Geometry check sheet. Reference: the model listing, model coordinates, mm. A direction names the side the tool comes from. Coordinates: 2 decimals unless noted, no trailing zeros. Order: outer loops, then holes, each group sorted by start corner. A loop starts at its lowest first (then second) coordinate and runs counter-clockwise, first axis right, second up. Notation, with made-up numbers: (-1.5, 61) - (39.5, 61) arc R18 cw to (39.5, 95) - close; hole circle Ø3 at (-36, 73.5). An arc over 180 degrees is marked (long way). Return JSON: item names as keys, results as strings. Group by question number.
Item 1: Draft check along Z on faces 1 (the flat face through (-1, -18.7, 15.3)), 2 (the flat face through (-3, -21, 15)), 3 (the cylindrical face through (19.783, -0.221, 28.686)). Enter one of: pulls with the +Z half, pulls with the -Z half, needs draft (parallel to the pull), parting line crosses it, or undercut.
Item 2: Section check B-B on x = 9. Enter the section's corners in (y, z), then the cut area to 3 significant figures.
Item 3: Section check A-A on z = 7.5. Enter the section's corners in (x, y), then the cut area to 3 significant figures.
Item 4: Section check C-C on y = 0. Enter the section's corners in (x, z).
Item 5: Tool access check on faces 4 (the flat face through (-13, -11, 37)), 5 (the flat face through (18.6, -5.6, 18.6)), 6 (the flat face through (1, -18.7, 15.3)), 7 (the cylindrical face through (19.783, -7.221, 21.686)), 8 (the flat face through (5, -25, 6)). Record the directions out of +Z, -Z, +X, -X, +Y, -Y that give a thin tool (end or side, any length) a straight path to the whole face; none if there is none.
Item 6: Gauge pin test, flat ends, axial feed: pin 1 (1 mm diameter, centred on x = -8, z = 9.5, fed in from +Y); pin 2 (3 mm diameter, centred on y = -24.5, z = 8.5, fed in from -X); pin 3 (3 mm diameter, centred on y = 1, z = 25.5, fed in from -X); pin 4 (6 mm diameter, centred on x = -13, y = -17, fed in from +Z). Record the tip position at first contact, or that the pin passes through.
Item 7: Scan lines: probe 1 along Y at (x, z) = (15, 13); probe 2 along Y at (x, z) = (14, 24); probe 3 along X at (y, z) = (1.5, 30). Record each from-to range of solid material in increasing order.
Item 8: Section check D-D on x = 2.5. Enter the section's corners in (y, z), then the cut area to 3 significant figures.
from build123d import *

# Parameters (mm, degrees)
BOSS_EXTRUDE1_DEPTH      = 40
EXTRUDE_START            = -25
SKETCH_5_W               = 10
SKETCH_5_H               = 28
EXTRUDE_2_DEPTH          = 15
CUT_EXTRUDE1_DEPTH       = 53.39274759
CUT_EXTRUDE1_DEPTH_BACK  = 53.39274759
SKETCH2_R                = 15
SKETCH5_R                = 11
CUT_EXTRUDE3_DEPTH       = 10
SKETCH7_W                = 6.152946469
SKETCH7_H                = 22
CUT_EXTRUDE9_DEPTH       = 10
SKETCH_2_W               = 5
SKETCH_2_H               = 14
CUT_EXTRUDE_2_DEPTH      = 20
CUT_EXTRUDE_6_DEPTH      = 51.368641203
CUT_EXTRUDE_6_DEPTH_BACK = 51.368641203
SKETCH_7_R               = 1.85
SKETCH6_W                = 2
SKETCH6_H                = 28
CUT_EXTRUDE8_DEPTH       = 53.392747702
CUT_EXTRUDE10_REACH      = 63.871
SKETCH8_R                = 3
CUT_EXTRUDE11_REACH      = 61.843
SKETCH13_R               = 3.25
SKETCH14_W               = 40
SKETCH14_H               = 38
SKETCH14_R               = 3
SKETCH14_R_2             = 1.7
BOSS_EXTRUDE2_DEPTH      = 2
CIRPATTERN1_START        = 10
CIRPATTERN1_OUTLINE_R    = 3.25
CIRPATTERN1_DEPTH        = 8.6
CIRPATTERN1_START_2      = 18.6
CIRPATTERN1_2_OUTLINE_R  = 1.7
CIRPATTERN1_2_DEPTH      = 2.4
CIRPATTERN2_START        = 15.6
CIRPATTERN2_OUTLINE_R    = 3.25
CIRPATTERN2_DEPTH        = 3
CIRPATTERN2_START_2      = 18.6
CIRPATTERN2_2_OUTLINE_R  = 1.7
CIRPATTERN2_2_DEPTH      = 2.4
CHAMFER1_SIZE            = 4


with BuildPart() as part:
    # Sketch1 → Boss-Extrude1 (new body)
    with BuildSketch(Plane.XY):
        with BuildLine():
            Line((0, 19), (19, 19))
            Line((19, 19), (19, -19))
            Line((19, -19), (0, -19))
            ThreePointArc((0, -19), (-19, 0), (0, 19))
        make_face()
    extrude(amount=BOSS_EXTRUDE1_DEPTH)

    # 草圖5 → 填料-伸長2 (add)
    with BuildSketch(Plane.XY.offset(40).offset(EXTRUDE_START)):
        with Locations((0, -14)):
            Rectangle(SKETCH_5_W, SKETCH_5_H)
    extrude(amount=-EXTRUDE_2_DEPTH)

    # Sketch2 → Cut-Extrude1 (cut, two sides: drawn at the far end of the back side and taken through both)
    with BuildSketch(Plane.XY.offset(40).offset(-CUT_EXTRUDE1_DEPTH_BACK)):
        Circle(SKETCH2_R)
    extrude(amount=CUT_EXTRUDE1_DEPTH + CUT_EXTRUDE1_DEPTH_BACK, mode=Mode.SUBTRACT)

    # Sketch5 → Cut-Extrude3 (cut)
    with BuildSketch(Plane(origin=(-19, 0, 0), x_dir=(0, 1, 0), z_dir=(-1, 0, 0))):
        with Locations((0, -34)):
            Circle(SKETCH5_R)
    extrude(amount=-CUT_EXTRUDE3_DEPTH, mode=Mode.SUBTRACT)

    # Sketch7 → Cut-Extrude9 (cut)
    with BuildSketch(Plane.ZY.offset(19)):
        with Locations((37.076473234, 0)):
            Rectangle(SKETCH7_W, SKETCH7_H)
    extrude(amount=-CUT_EXTRUDE9_DEPTH, mode=Mode.SUBTRACT)

    # 草圖2 → 除料-伸長2 (cut)
    with BuildSketch(Plane.XY.offset(40)):
        with Locations((13.1, 0)):
            Rectangle(SKETCH_2_W, SKETCH_2_H)
    extrude(amount=-CUT_EXTRUDE_2_DEPTH, mode=Mode.SUBTRACT)

    # 草圖7 → 除料-伸長6 (cut, two sides: drawn at the far end of the back side and taken through both)
    with BuildSketch(Plane(origin=(0, -5, 0), x_dir=(0, 0, 1), z_dir=(-1, 0, 0)).offset(-CUT_EXTRUDE_6_DEPTH_BACK)):
        with Locations(Location((7.5, -18, 0), (0, 0, 90))):
            Circle(SKETCH_7_R)
    extrude(amount=CUT_EXTRUDE_6_DEPTH + CUT_EXTRUDE_6_DEPTH_BACK, mode=Mode.SUBTRACT)

    # Sketch6 → Cut-Extrude8 (cut, through all)
    with BuildSketch(Plane.XY):
        with Locations((0, -14)):
            Rectangle(SKETCH6_W, SKETCH6_H)
    extrude(amount=CUT_EXTRUDE8_DEPTH, mode=Mode.SUBTRACT)

    # Sketch8 → Cut-Extrude10 (cut, up to next)
    with BuildSketch(Plane(origin=(19, 0, 0), x_dir=(0, 0, -1), z_dir=(1, 0, 0)), mode=Mode.PRIVATE) as cut_extrude10_sk1:
        with Locations((-20, 0)):
            Circle(SKETCH8_R)
    cut_extrude10_tool1 = extrude(cut_extrude10_sk1.sketch, amount=-CUT_EXTRUDE10_REACH, mode=Mode.PRIVATE) & part.part
    add(cut_extrude10_tool1.solids().sort_by_distance((19, 0, 20))[0], mode=Mode.SUBTRACT)

    # Sketch12 → CBORE for M3 SHCS1 (revolve, cut)
    with BuildSketch(Plane(origin=(15.6, 7, 20), x_dir=(0, 0, 1), z_dir=(0, 1, 0))):
        Polygon((0, 0), (0, 3.4), (1.7, 3.4), (1.7, 3), (3.25, 3), (3.25, 0), align=None)
    revolve(axis=Axis((9.25, 7, 20), (1, 0, 0)), mode=Mode.SUBTRACT)

    # Sketch13 → Cut-Extrude11 (cut, up to next)
    with BuildSketch(Plane(origin=(15.6, 0, 0), x_dir=(0, 0, -1), z_dir=(1, 0, 0)), mode=Mode.PRIVATE) as cut_extrude11_sk1:
        with Locations(Location((-20, 7, 0), (0, 0, 180))):
            Circle(SKETCH13_R)
    cut_extrude11_tool1 = extrude(cut_extrude11_sk1.sketch, amount=-CUT_EXTRUDE11_REACH, mode=Mode.PRIVATE) & part.part
    add(cut_extrude11_tool1.solids().sort_by_distance((15.6, 7, 20))[0], mode=Mode.SUBTRACT)

    # Sketch14 → Boss-Extrude2 (add)
    with BuildSketch(Plane(origin=(19, 0, 0), x_dir=(0, 0, -1), z_dir=(1, 0, 0))):
        with Locations((-20, 0)):
            Rectangle(SKETCH14_W, SKETCH14_H)
        with Locations((-20, 0)):
            Circle(SKETCH14_R, mode=Mode.SUBTRACT)
        with Locations(Location((-20, 7, 0), (0, 0, 180))):
            Circle(SKETCH14_R_2, mode=Mode.SUBTRACT)
    extrude(amount=BOSS_EXTRUDE2_DEPTH)

    # CirPattern1: read off the stored shape, not the designer's step
    # CirPattern1 outline → CirPattern1 (cut)
    with BuildSketch(Plane.YZ.offset(CIRPATTERN1_START)):
        with Locations((0, 13)):
            Circle(CIRPATTERN1_OUTLINE_R)
        with Locations((-7, 20)):
            Circle(CIRPATTERN1_OUTLINE_R)
    extrude(amount=CIRPATTERN1_DEPTH, mode=Mode.SUBTRACT)

    # CirPattern1 2 outline → CirPattern1 2 (cut)
    with BuildSketch(Plane.YZ.offset(CIRPATTERN1_START_2)):
        with Locations((0, 13)):
            Circle(CIRPATTERN1_2_OUTLINE_R)
        with Locations((-7, 20)):
            Circle(CIRPATTERN1_2_OUTLINE_R)
    extrude(amount=CIRPATTERN1_2_DEPTH, mode=Mode.SUBTRACT)

    # CirPattern2: read off the stored shape, not the designer's step
    # CirPattern2 outline → CirPattern2 (cut)
    with BuildSketch(Plane.YZ.offset(CIRPATTERN2_START)):
        with Locations((0, 27)):
            Circle(CIRPATTERN2_OUTLINE_R)
    extrude(amount=CIRPATTERN2_DEPTH, mode=Mode.SUBTRACT)

    # CirPattern2 2 outline → CirPattern2 2 (cut)
    with BuildSketch(Plane.YZ.offset(CIRPATTERN2_START_2)):
        with Locations((0, 27)):
            Circle(CIRPATTERN2_2_OUTLINE_R)
    extrude(amount=CIRPATTERN2_2_DEPTH, mode=Mode.SUBTRACT)

    # Chamfer1
    chamfer1_edges = [part.edges().sort_by_distance(p)[0] for p in [
        (21, -19, 20),
        (21, 19, 20),
        (-3, -28, 15),
        (-3, -28, 0),
        (3, -28, 15),
        (3, -28, 0),
    ]]
    chamfer(chamfer1_edges, length=CHAMFER1_SIZE)


solid = part.part
Computed:
{
 "1": {"face 1": "needs draft", "face 2": "pulls with the +Z half", "face 3": "undercut"},
 "2": {"outline": "(-19, 0) - (-12, 0) - (-12, 40) - (-19, 40) - close; (12, 0) - (19, 0) - (19, 40) - (12, 40) - close", "area": "560 mm²"},
 "3": {"outline": "(-5, -28) - (-1, -28) - (-1, -24.85) - (-5, -24.85) - close; (-5, -21.15) - (-1, -21.15) - (-1, -14.97) arc R15 cw (long way) to (1, -14.97) - (1, -21.15) - (5, -21.15) - (5, -19) - (17, -19) - (21, -15) - (21, 15) - (17, 19) - (0, 19) arc R19 ccw to (-5, -18.33) - close; (1, -28) - (5, -28) - (5, -24.85) - (1, -24.85) - close", "area": "678 mm²"},
 "4": {"outline": "(-19, 0) - (-15, 0) - (-15, 23) - (-19, 23) - close; (15, 0) - (21, 0) - (21, 11.3) - (18.6, 11.3) - (18.6, 9.75) - (15, 9.75) - close; (15, 16.25) - (18.6, 16.25) - (18.6, 14.7) - (21, 14.7) - (21, 17) - (15, 17) - close; (15.6, 23) - (21, 23) - (21, 25.3) - (18.6, 25.3) - (18.6, 23.75) - (15.6, 23.75) - close; (15.6, 30.25) - (18.6, 30.25) - (18.6, 28.7) - (21, 28.7) - (21, 40) - (15.6, 40) - close"},
 "5": {"face 4": "+Z, -X", "face 5": "none", "face 6": "+Z, -Z, -Y", "face 7": "+X", "face 8": "+Z, -Z, +X, -Y"},
 "6": {"pin 1": "stops at y = 17.46", "pin 2": "stops at x = -5", "pin 3": "stops at x = 15.6", "pin 4": "stops at z = 40"},
 "7": {"probe 1": "y = -19 to -3.25, 3.25 to 19", "probe 2": "y = -19 to -7, 7 to 19", "probe 3": "x = 15.6 to 21"},
 "8": {"outline": "(-28, 4) - (-24, 0) - (-14.79, 0) - (-14.79, 40) - (-19, 40) - (-19, 15) - (-24, 15) - (-28, 11) - close; (14.79, 0) - (19, 0) - (19, 40) - (14.79, 40) - close; hole circle Ø3.7 at (-23, 7.5)", "area": "445 mm²"}
}
